```python
from build123d import *

# Parameters (mm, degrees)
SKETCH1_W                                    = 58
SKETCH1_H                                    = 35
BOSS_EXTRUDE1_DEPTH                          = 2
CSK_FOR_ST2_2_CROSS_RECESSED_CTSK_HE_2_COUNT = 2
CSK_FOR_ST2_2_CROSS_RECESSED_CTSK_HE_2_PITCH = 20
CSK_FOR_ST2_2_CROSS_RECESSED_CTSK_HE_3_COUNT = 2
CSK_FOR_ST2_2_CROSS_RECESSED_CTSK_HE_3_PITCH = 39.8
CSK_FOR_ST2_2_CROSS_RECESSED_CTSK_HE_4_COUNT = 2
CSK_FOR_ST2_2_CROSS_RECESSED_CTSK_HE_4_PITCH = 44.102607633
CSK_FOR_ST2_2_CROSS_RECESSED_CTSK_HE_5_COUNT = 2
CSK_FOR_ST2_2_CROSS_RECESSED_CTSK_HE_5_PITCH = 14
CHAMFER1_SIZE                                = 2


with BuildPart() as part:
    # Sketch1 → Boss-Extrude1 (new body)
    with BuildSketch(Plane(origin=(0, 0, 0), x_dir=(1, 0, 0), z_dir=(0, 1, 0))):
        Rectangle(SKETCH1_W, SKETCH1_H)
    extrude(amount=BOSS_EXTRUDE1_DEPTH)

    # Sketch3 → CSK for ST2.2 Cross recessed CTSK head tapping screws1 (revolve, cut)
    with BuildSketch(Plane(origin=(-23, 2, -12.5), x_dir=(0, 0, 1), z_dir=(1, 0, 0))):
        Polygon((0, 0), (0, 2), (1.75, 2), (1.75, 0.6), (2.35, 0), align=None)
    csk_for_st2_2_cross_recessed_ctsk_head_t = revolve(axis=Axis((-23, 8.35, -12.5), (0, -1, 0)), mode=Mode.SUBTRACT)

    # CSK for ST2.2 Cross recessed CTSK he 2: CSK for ST2.2 Cross recessed CTSK head tapping screws1 ×2
    with Locations(*[(i * CSK_FOR_ST2_2_CROSS_RECESSED_CTSK_HE_2_PITCH, 0, 0) for i in range(1, CSK_FOR_ST2_2_CROSS_RECESSED_CTSK_HE_2_COUNT)]):
        add(csk_for_st2_2_cross_recessed_ctsk_head_t, mode=Mode.SUBTRACT)

    # CSK for ST2.2 Cross recessed CTSK he 3: CSK for ST2.2 Cross recessed CTSK head tapping screws1 ×2
    with Locations(*[(i * CSK_FOR_ST2_2_CROSS_RECESSED_CTSK_HE_3_PITCH, 0, 0) for i in range(1, CSK_FOR_ST2_2_CROSS_RECESSED_CTSK_HE_3_COUNT)]):
        add(csk_for_st2_2_cross_recessed_ctsk_head_t, mode=Mode.SUBTRACT)

    # CSK for ST2.2 Cross recessed CTSK he 4: CSK for ST2.2 Cross recessed CTSK head tapping screws1 ×2
    with Locations(*[Vector(0.9024409697382602, 0, 0.4308135282670086) * (i * CSK_FOR_ST2_2_CROSS_RECESSED_CTSK_HE_4_PITCH) for i in range(1, CSK_FOR_ST2_2_CROSS_RECESSED_CTSK_HE_4_COUNT)]):
        add(csk_for_st2_2_cross_recessed_ctsk_head_t, mode=Mode.SUBTRACT)

    # CSK for ST2.2 Cross recessed CTSK he 5: CSK for ST2.2 Cross recessed CTSK head tapping screws1 ×2
    with Locations(*[(0, 0, i * CSK_FOR_ST2_2_CROSS_RECESSED_CTSK_HE_5_PITCH) for i in range(1, CSK_FOR_ST2_2_CROSS_RECESSED_CTSK_HE_5_COUNT)]):
        add(csk_for_st2_2_cross_recessed_ctsk_head_t, mode=Mode.SUBTRACT)

    # Chamfer1
    chamfer1_edges = [part.edges().sort_by_distance(p)[0] for p in [
        (29, 1, 17.5),
        (-29, 1, 17.5),
        (-29, 1, -17.5),
        (29, 1, -17.5),
    ]]
    chamfer(chamfer1_edges, length=CHAMFER1_SIZE)


solid = part.part
```
For this review, take the finished solid that the model builds, in its own axes (mm). Round coordinates to 2 decimals unless told otherwise and drop trailing zeros. Order: outer loops, then holes, each group sorted by start corner. A loop starts at its lowest first (then second) coordinate and runs counter-clockwise, first axis right, second up.
Q1. We need section A-A, the plane z = -12.5. Give the boundary of the cut face in (x, y), plus the area to 3 significant figures.
Findings below:
outline: (-29, 0) - (-24.75, 0) - (-24.75, 1.4) - (-25.35, 2) - (-29, 2) - close; (-21.25, 0) - (-4.75, 0) - (-4.75, 1.4) - (-5.35, 2) - (-20.65, 2) - (-21.25, 1.4) - close; (-1.25, 0) - (15.05, 0) - (15.05, 1.4) - (14.45, 2) - (-0.65, 2) - (-1.25, 1.4) - close; (18.55, 0) - (29, 0) - (29, 2) - (19.15, 2) - (18.55, 1.4) - close
area: 93.9 mm2
Q2. We need section C-C, the plane z = 6.5. Give the boundary of the cut face in (x, y).
Findings below:
outline: (-29, 0) - (15.05, 0) - (15.05, 1.4) - (14.45, 2) - (-29, 2) - close; (18.55, 0) - (29, 0) - (29, 2) - (19.15, 2) - (18.55, 1.4) - close
Q3. We need section D-D, the plane x = 16.8. Give the boundary of the cut face in (y, z), plus the area to 3 significant figures.
Findings below:
outline: (0, -17.5) - (2, -17.5) - (2, -14.85) - (1.4, -14.25) - (0, -14.25) - close; (0, -10.75) - (1.4, -10.75) - (2, -10.15) - (2, 4.15) - (1.4, 4.75) - (0, 4.75) - close; (0, 8.25) - (1.4, 8.25) - (2, 8.85) - (2, 17.5) - (0, 17.5) - close
area: 55.3 mm2
Q4. Mouldability with a two-part tool opening along X and no side actions: class faces 1 (the flat face through (-28, 1, -16.5)), 2 (the cylindrical face through (15.065, 0.71, -12.728)), 3 (the cylindrical face through (-24.735, 0.71, 1.272)), 4 (the flat face through (0, 1, 17.5)) as pulls with the +X half, pulls with the -X half, needs draft (parallel to the pull), parting line crosses it, or undercut.
Findings below:
face 1: pulls with the -X half
face 2: undercut
face 3: undercut
face 4: needs draft
Q5. Insertion check: P1, Ø4, axis at x = -23, z = 1.5, coming from the +Y side; P2, Ø3, axis at x = -23, z = -12.5, coming from the -Y side. Each pin has a flat end and moves straight along its axis. Give the tip position at first contact, or say it passes through.
Findings below:
P1: stops at y = 1.65
P2: passes through
Q6. We need section B-B, the plane x = -3. Give the boundary of the cut face in (y, z).
Findings below:
outline: (0, -17.5) - (2, -17.5) - (2, -14.85) - (1.4, -14.25) - (0, -14.25) - close; (0, -10.75) - (1.4, -10.75) - (2, -10.15) - (2, 17.5) - (0, 17.5) - close
Q7. Wall thickness on line 1 (X direction, y = 0.75, z = -12.5); line 2 (Z direction, x = -25, y = 1.95); line 3 (Z direction, x = -21.5, y = 1.2): over which ranges is each line inside the solid? List them lowest first.
Findings below:
line 1: x = -29 to -24.75, -21.25 to -4.75, -1.25 to 15.05, 18.55 to 29
line 2: z = -17.5 to -13.64, -11.36 to 0.36, 2.64 to 17.5
line 3: z = -17.5 to -13.4, -11.6 to 0.6, 2.4 to 17.5
